CAD build for the part. Positions are in the model's coordinates, mm. Round coordinates to 2 decimals unless told otherwise and drop trailing zeros. Write each loop counter-clockwise with the first axis right and the second up, starting at its lowest first coordinate (ties: lowest second). Pieces come first, ordered by that corner, then holes. Notation, with made-up numbers: (25.5, 32) - (83.5, 32) arc R26 ccw to (83.5, 65) - close; hole circle Ø4 at (39, 5). An arc over 180 degrees is marked (long way). Use one line per item in the form item = value. Start each with the question number.
Item 1: Pin check, flat tip, straight feed: pin 1 (6 mm diameter, centred on x = 359, z = -180.5, fed in from +Y). Stop position of the tip, or through.
Item 2: Drill centre lines: L1, parallel to Y at x = 235, z = -210.5; L2, parallel to Y at x = 255, z = -238.5. Where is each one in solid material? Low to high.
Item 3: Band-saw the part on A-A, the plane x = 209. List the corners of the cut face in (y, z) (3 decimals), and give its area (3 significant figures).
Item 4: Band-saw the part on C-C, the plane z = -212. List the corners of the cut face in (x, y) (3 decimals).
Item 5: Band-saw the part on B-B, the plane z = -93. List the corners of the cut face in (x, y) (3 decimals), and give its area (3 significant figures).
Autodesk Inventor part; units mm, degrees
ref_plane "YZ Plane" through (0, 0, 0) normal (1, 0, 0) x (0, 1, 0)
ref_plane "XZ Plane" through (0, 0, 0) normal (0, 1, 0) x (-1, 0, 0)
ref_plane "XY Plane" through (0, 0, 0) normal (0, 0, 1) x (1, 0, 0)
sketch "Sketch2" plane through (0, 0, 0) normal (1, 0, 0) x (0, 1, 0)
  line L0 (0, 0) -> (152.4, 0)
  line L1 (152.4, 0) -> (152.4, -295.275)
  line L2 (152.4, -295.275) -> (0, -295.275)
  line L3 (0, -295.275) -> (0, 0)
  line L4 (152.4, -295.275) -> (139.7, 0)
  line L5 (0, -9.525) -> (6.35, -9.525)
  line L6 (6.35, -9.525) -> (6.35, -15.875)
  line L7 (6.35, -15.875) -> (0, -15.875)
  line L8 (0, -15.875) -> (0, -9.525)
  point P0 (0, -15.875)
  dimension "d4" = 152.4
  dimension "d5" = 295.275
  dimension "d6" = 12.7
  dimension "d7" = 6.35
  dimension "d8" = 6.35
  dimension "d9" = 9.525
extrude "Extrusion2" add sketch "Sketch2" along normal blind 447.675 contours L0 L4 L2 L3 L7 L6 L5
Determined:
q1.pin_1 = 147.59
q2.L1 = 0 to 148.75
q2.L2 = 0 to 149.96
q3.outline = (0, -295.275) - (152.4, -295.275) - (139.7, 0) - (0, 0) - (0, -9.525) - (6.35, -9.525) - (6.35, -15.875) - (0, -15.875) - close
q3.area = 43,100 mm²
q4.outline = (0, 0) - (447.675, 0) - (447.675, 148.818) - (0, 148.818) - close
q5.outline = (0, 0) - (447.675, 0) - (447.675, 143.7) - (0, 143.7) - close
q5.area = 64,300 mm²
